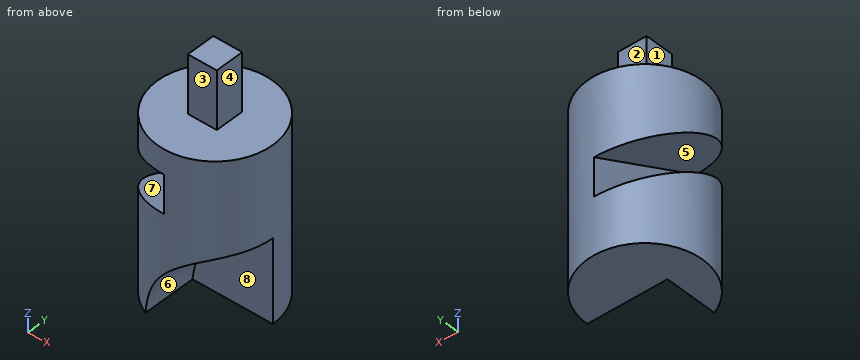
from build123d import *

# Parameters (mm, degrees)
F0_W     = 25.4
F0_H     = 76.2
F3_DEPTH = 58.42
F4_W     = 12.7
F4_H     = 12.7
F5_DEPTH = 25.4
F6_R     = 40.643977
F7_DEPTH = 87.884


with BuildPart() as f1:
    # F0 (on Front) → F1 (revolve)
    with BuildSketch(Plane.XZ):
        with Locations((12.7, -7.62)):
            Rectangle(F0_W, F0_H)
    revolve(axis=Axis((0, 0, -7.62), (0, 0, -1)))

    # F2 (on Right) → F3 (cut)
    with BuildSketch(Plane.YZ):
        Polygon((45.269145, -13.24631), (-37.608135, 25.4), (-44.048837, 11.587869), (38.828442, -27.058441), align=None)
    extrude(amount=-F3_DEPTH, mode=Mode.SUBTRACT)

    # F4 (on face) → F5 (join)
    with BuildSketch(Plane.XY.offset(30.48)):
        Rectangle(F4_W, F4_H)
    extrude(amount=F5_DEPTH)

    # F6 (on Front) → F7 (cut)
    with BuildSketch(Plane.XZ):
        with Locations((30.542457, -49.467545)):
            Circle(F6_R)
    extrude(amount=F7_DEPTH, mode=Mode.SUBTRACT)


solid = f1.part
Read the model definition and answer for the solid it produces. Units are mm, in the model's axes. Face numbers are marked on the shaded views. A direction names the side the tool comes from. Coordinates: 2 decimals unless noted, no trailing zeros. Order: outer loops, then holes, each group sorted by start corner. A loop starts at its lowest first (then second) coordinate and runs counter-clockwise, first axis right, second up. Notation, with made-up numbers: M 42,45 L 87,45 A14 cw 87,59 Z; hole C -20,-20.5 d8. An arc over 180 degrees is marked long. Put each result on its own line as item: value. Start each with the question number.
Item 1: Consider probe 1 along X at (y, z) = (-1, 5.5); probe 2 along Y at (x, z) = (-5.5, -1.5); probe 3 along X at (y, z) = (2, 45.5). Determine where each line is inside the solid, lowest interval first. Write a range as [from, to].
Item 2: Section B-B, the plane y = -3 is taken. Determine the outline of the cut face in (x, z), plus the area to 3 significant figures.
Item 3: Section C-C, the plane z = -14 is taken. Determine the outline of the cut face in (x, y).
Item 4: The mould has two halves that part along Z. Classify the marked faces 5, 6, 7 and 8: +Z half, -Z half, draft (parallel to the pull), parting line (faces both ways), or undercut.
Item 5: Given pin 1 Ø6.5 at (x, z) = (-3, 47.5) entering from -Y; pin 2 Ø8 at (x, z) = (-6, -2) entering from +Y; pin 3 Ø2 at (y, z) = (4.5, -25.5) entering from -X, each flat-ended and moving along its own axis, determine where each tip first touches the part or whether it passes through.
Item 6: For the marked faces 1, 2, 3 and 4, determine the directions among +Z, -Z, +X, -X, +Y, -Y from which every point of the face is accessible in a straight line to the end or side of a thin tool.
Item 7: Section D-D, the plane x = 16 is taken. Determine the outline of the cut face in (y, z).
Item 8: Section A-A, the plane x = -16 is taken. Determine the outline of the cut face in (y, z).
Computed:
1. probe 1: x = [0, 25.38]
1. probe 2: y = [-24.8, -15.98], [20.08, 24.8]
1. probe 3: x = [-6.35, 6.35]
2. outline: M -25.22,-45.72 L -9.93,-45.72 A40.64 cw 25.22,-9.17 L 25.22,30.48 L 6.35,30.48 L 6.35,55.88 L -6.35,55.88 L -6.35,30.48 L -25.22,30.48 L -25.22,9.26 L 0,9.26 L 0,-7.55 L -25.22,-7.55 Z
2. area: 2,790 mm2
3. outline: M -22.98,10.82 A25.4 ccw 10.69,-23.04 L 10.69,0 L 25.4,0 A25.4 ccw 0,25.4 L 0,10.82 Z
4. face 5: undercut
4. face 6: -Z half
4. face 7: undercut
4. face 8: draft
5. pin 1: stops at y = -6.35
5. pin 2: stops at y = 25.32
5. pin 3: stops at x = -25.16
6. face 1: +Z, -X, +Y, -Y
6. face 2: +Z, +X, -X, +Y
6. face 3: +Z, +X, -X, -Y
6. face 4: +Z, +X, +Y, -Y
7. outline: M -19.73,-11.51 L 0,-11.51 L 0,-45.72 L 19.73,-45.72 L 19.73,30.48 L -19.73,30.48 Z
8. outline: M -19.73,-45.72 L 19.73,-45.72 L 19.73,-18.15 L -19.73,0.25 Z; M -19.73,17.06 L 19.73,-1.34 L 19.73,30.48 L -19.73,30.48 Z
